Can you work these out from the model? Positions are in its coordinate system, mm. Face numbers are marked on the shaded views. Round coordinates to 2 decimals unless told otherwise and drop trailing zeros. Loops run counter-clockwise (first coordinate to the right, second up) from the corner with the lowest first, then second, coordinate; pieces in that order, holes last.
from build123d import *

# Parameters (mm, degrees)
SKETCH1_R           = 0.9906
SKETCH1_R_2         = 1.6
SKETCH1_R_3         = 3.5
BOSS_EXTRUDE2_DEPTH = 3.175


with BuildPart() as part:
    # Sketch1 → Boss-Extrude2 (new body)
    with BuildSketch(Plane.XY):
        with BuildLine():
            Line((0, 0), (37.166699296, 0))
            Line((37.166699296, 0), (37.166699296, 6.5))
            ThreePointArc((37.166699296, 6.5), (30.666699296, 13), (37.166699296, 19.5))
            Line((37.166699296, 19.5), (37.166699296, 30))
            Line((37.166699296, 30), (0, 30))
            Line((0, 30), (0, 0))
        make_face()
        with Locations((25.169778966, 20.933400182)):
            Circle(SKETCH1_R, mode=Mode.SUBTRACT)
        with Locations((16, 24.5)):
            Circle(SKETCH1_R_2, mode=Mode.SUBTRACT)
        with Locations((24, 15)):
            Circle(SKETCH1_R_2, mode=Mode.SUBTRACT)
        with Locations(Location((16, 5.5, 0), (0, 0, 180))):
            Circle(SKETCH1_R_2, mode=Mode.SUBTRACT)
        with Locations(Location((8, 15, 0), (0, 0, 180))):
            Circle(SKETCH1_R_2, mode=Mode.SUBTRACT)
        with Locations((16, 15)):
            Circle(SKETCH1_R_3, mode=Mode.SUBTRACT)
    extrude(amount=BOSS_EXTRUDE2_DEPTH)


solid = part.part
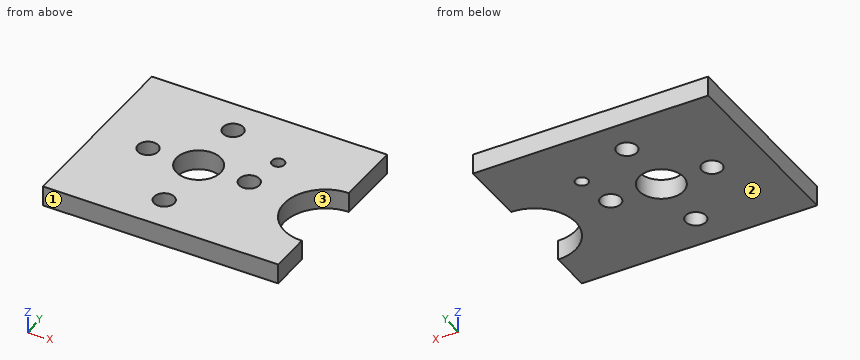
(1) If we section it at B-B, the plane y = 24.5: List the corners of the cut face in (x, z) for me (3 decimals), then the cut area to 3 significant figures.
Worked answers:
outline: (0, 0) - (14.4, 0) - (14.4, 3.175) - (0, 3.175) - close; (17.6, 0) - (37.167, 0) - (37.167, 3.175) - (17.6, 3.175) - close
area: 108 mm2
(2) If I drill on line 1 (Y direction, x = 16, z = 2); line 2 (X direction, y = 21, z = 1.35); line 3 (Y direction, x = 24, z = 1.8), over which ranges is the centre line in solid material (lowest first)?
Worked answers:
line 1: y = 0 to 3.9, 7.1 to 11.5, 18.5 to 22.9, 26.1 to 30
line 2: x = 0 to 24.18, 26.16 to 37.17
line 3: y = 0 to 13.4, 16.6 to 30
(3) If we section it at A-A, the plane x = 16: List the corners of the cut face in (y, z) for me (3 decimals), then the cut area to 3 significant figures.
Worked answers:
outline: (0, 0) - (3.9, 0) - (3.9, 3.175) - (0, 3.175) - close; (7.1, 0) - (11.5, 0) - (11.5, 3.175) - (7.1, 3.175) - close; (18.5, 0) - (22.9, 0) - (22.9, 3.175) - (18.5, 3.175) - close; (26.1, 0) - (30, 0) - (30, 3.175) - (26.1, 3.175) - close
area: 52.7 mm2
(4) If we section it at D-D, the plane y = 15: List the corners of the cut face in (x, z) for me (3 decimals).
Worked answers:
outline: (0, 0) - (6.4, 0) - (6.4, 3.175) - (0, 3.175) - close; (9.6, 0) - (12.5, 0) - (12.5, 3.175) - (9.6, 3.175) - close; (19.5, 0) - (22.4, 0) - (22.4, 3.175) - (19.5, 3.175) - close; (25.6, 0) - (30.982, 0) - (30.982, 3.175) - (25.6, 3.175) - close
(5) If we mould it in two halves opening along Y, with no side actions, what happens to the marked faces 1, 2 and 3? For each: released by +Y, released by -Y, zero draft, split by the parting line, or undercut.
Worked answers:
face 1: released by -Y
face 2: zero draft
face 3: undercut
(6) If we section it at C-C, the plane x = 8: List the corners of the cut face in (y, z) for me (3 decimals), then the cut area to 3 significant figures.
Worked answers:
outline: (0, 0) - (13.4, 0) - (13.4, 3.175) - (0, 3.175) - close; (16.6, 0) - (30, 0) - (30, 3.175) - (16.6, 3.175) - close
area: 85.1 mm2
(7) Will this pin go through, and if not, where does the flat tip stop? P1, Ø1.9, axis at x = 8, y = 15, coming from the -Z side.
Worked answers:
P1: passes through
